Work out the finished part from the listing and answer in its coordinate system (mm). A direction names the side the tool comes from. Give positions to 0.01 mm unless a question says otherwise; leave off trailing zeros. Loops run counter-clockwise (first coordinate to the right, second up) from the corner with the lowest first, then second, coordinate; pieces in that order, holes last. Notation, with made-up numbers: (40, 55.25) - (55, 55.25) arc R16 cw to (55, 86.25) - close; hole circle Ø11 at (39, 26.25). An arc over 180 degrees is marked (long way). Use CSV: the item, a comma, the result in double quotes.
from build123d import *

# Parameters (mm, degrees)
F0_W        = 63.1147548556
F0_H        = 73.1557384133
F1_DEPTH    = 7
F2_R        = 15.8223055834
F3_DEPTH    = 3
F4_T        = -2.5
F5_T1_DEPTH = 32


# Not quite as in the source:
# - a fillet or chamfer that OpenCascade refuses, or shapes differently, is made with other operations: its cross-section is extruded or revolved along the edge and cut away or added


with BuildPart() as f1:
    # F0 (on Front) → F1 (new body)
    with BuildSketch(Plane.XZ):
        Rectangle(F0_W, F0_H)
    extrude(amount=F1_DEPTH)

    # F2 (on face) → F3 (join)
    with BuildSketch(Plane.XZ.offset(7)):
        Circle(F2_R)
    extrude(amount=F3_DEPTH)

    # F4
    f4_openings = [f1.faces().sort_by_distance(p)[0] for p in [
        (0, -3.5, 36.577869),
    ]]
    offset(amount=F4_T, openings=f4_openings, kind=Kind.INTERSECTION)

    # F5: fillet of radius 5 on 4 edges, made by hand

    # F5_s2 → F5_t1 (cut)
    with BuildSketch(Plane.XZ.offset(-12.5)):
        with BuildLine():
            ThreePointArc((31.5573774278, 31.5778692067), (30.0929113337, 35.1134031126), (26.5573774278, 36.5778692067))
            Line((26.5573774278, 36.5778692067), (31.5573774278, 36.5778692067))
            Line((31.5573774278, 36.5778692067), (31.5573774278, 31.5778692067))
        make_face()
        with BuildLine():
            ThreePointArc((31.5573774278, -31.5778692067), (30.0929113337, -35.1134031126), (26.5573774278, -36.5778692067))
            Line((26.5573774278, -36.5778692067), (31.5573774278, -36.5778692067))
            Line((31.5573774278, -36.5778692067), (31.5573774278, -31.5778692067))
        make_face()
        with BuildLine():
            ThreePointArc((-31.5573774278, -31.5778692067), (-30.0929113337, -35.1134031126), (-26.5573774278, -36.5778692067))
            Line((-26.5573774278, -36.5778692067), (-31.5573774278, -36.5778692067))
            Line((-31.5573774278, -36.5778692067), (-31.5573774278, -31.5778692067))
        make_face()
        with BuildLine():
            ThreePointArc((-31.5573774278, 31.5778692067), (-30.0929113337, 35.1134031126), (-26.5573774278, 36.5778692067))
            Line((-26.5573774278, 36.5778692067), (-31.5573774278, 36.5778692067))
            Line((-31.5573774278, 36.5778692067), (-31.5573774278, 31.5778692067))
        make_face()
    extrude(amount=F5_T1_DEPTH, mode=Mode.SUBTRACT)


solid = f1.part
Item 1: For faces 5 (the flat face through (-14, -7, 9)), 6 (the flat face through (0, -2.5, 2)), 7 (the flat face through (0, -7.5, 0)), determine the directions among +Z, -Z, +X, -X, +Y, -Y from which every point of the face is accessible in a straight line to the end or side of a thin tool.
Determined:
face 5,"-Y"
face 6,"+Z"
face 7,"none"
Item 2: Find the intervals of material crossed by line 1 (X direction, y = -5.9, z = 0); line 2 (Z direction, x = 0, y = -6.6); line 3 (Y direction, x = -10.5, z = 3.5), in increasing order.
Determined:
line 1,"x = -31.56 to -13.32, 13.32 to 31.56"
line 2,"z = -36.58 to -13.32, 13.32 to 36.58"
line 3,"y = -10 to -7.5, -2.5 to 0"
Item 3: Given P1, Ø1, axis at x = -4, y = -3.5, coming from the +Z side, flat-ended and moving along its own axis, determine where the tip first touches the part or whether it passes through.
Determined:
P1,"stops at z = -34.08"
Item 4: A cutting plane is placed at A-A on x = 0. Determine the outline of the cut face in (y, z).
Determined:
outline,"(-10, -15.82) - (-7, -15.82) - (-7, -36.58) - (0, -36.58) - (0, 36.58) - (-2.5, 36.58) - (-2.5, -34.08) - (-4.5, -34.08) - (-4.5, -13.32) - (-7.5, -13.32) - (-7.5, 13.32) - (-4.5, 13.32) - (-4.5, 36.58) - (-7, 36.58) - (-7, 15.82) - (-10, 15.82) - close"
Item 5: A cutting plane is placed at B-B on z = -28. Determine the outline of the cut face in (x, y), and give its area (3 significant figures).
Determined:
outline,"(-31.56, -7) - (31.56, -7) - (31.56, 0) - (-31.56, 0) - close; hole (-29.06, -4.5) - (29.06, -4.5) - (29.06, -2.5) - (-29.06, -2.5) - close"
area,"326 mm²"
Item 6: A cutting plane is placed at C-C on z = 0. Determine the outline of the cut face in (x, y).
Determined:
outline,"(-31.56, -7) - (-15.82, -7) - (-15.82, -10) - (15.82, -10) - (15.82, -7) - (31.56, -7) - (31.56, 0) - (-31.56, 0) - close; hole (-29.06, -4.5) - (-13.32, -4.5) - (-13.32, -7.5) - (13.32, -7.5) - (13.32, -4.5) - (29.06, -4.5) - (29.06, -2.5) - (-29.06, -2.5) - close"
Item 7: The mould has two halves that part along X. Classify faces 1 (the flat face through (29.057, -3, 0)), 2 (the cylindrical face through (-3.43, -8.479, -15.446)), 3 (the cylindrical face through (-1.73, -5.98, 13.21)), 4 (the flat face through (0, -1, 36.578)): pulls with the +X half, pulls with the -X half, needs draft (parallel to the pull), parting line crosses it, or undercut.
Determined:
face 1,"undercut"
face 2,"parting line crosses it"
face 3,"undercut"
face 4,"needs draft"
Item 8: A cutting plane is placed at D-D on x = -23. Determine the outline of the cut face in (y, z), and give its area (3 significant figures).
Determined:
outline,"(-7, -36.58) - (0, -36.58) - (0, 36.58) - (-2.5, 36.58) - (-2.5, -34.08) - (-4.5, -34.08) - (-4.5, 36.58) - (-7, 36.58) - close"
area,"371 mm²"
